from build123d import *

# Parameters (mm, degrees)
SKETCH1_W            = 133.35
SKETCH1_H            = 76.2
BOSS_EXTRUDE1_DEPTH  = 3
M2_CLEARANCE_HOLE1_D = 2.6
SKETCH7_R            = 3.75
SKETCH7_R_2          = 1.665
BOSS_EXTRUDE2_DEPTH  = 5.5
CUT_EXTRUDE1_DEPTH   = 77.989711163
FILLET1_R            = 5
SKETCH9_R            = 2.25
CUT_EXTRUDE2_DEPTH   = 1


with BuildPart() as part:
    # Sketch1 → Boss-Extrude1 (new body)
    with BuildSketch(Plane(origin=(0, 0, 0), x_dir=(0, 0, -1), z_dir=(1, 0, 0))):
        Rectangle(SKETCH1_W, SKETCH1_H)
    extrude(amount=BOSS_EXTRUDE1_DEPTH)

    # M2 Clearance Hole1 (through all)
    with Locations(Plane(origin=(3, 0, 0), x_dir=(0, 0, -1), z_dir=(1, 0, 0))):
        with Locations((-45, -30.1), (-45, 30.1), (42, 30.1), (42, -30.1)):
            Hole(M2_CLEARANCE_HOLE1_D / 2)

    # Sketch7 → Boss-Extrude2 (add)
    # profile 1 of 4: a face of its own
    with BuildSketch(Plane(origin=(3, 0, 0), x_dir=(0, 0, -1), z_dir=(1, 0, 0))):
        with Locations((-30.23150301, -26.854999996)):
            Circle(SKETCH7_R)
        with Locations((-30.23150301, -26.854999996)):
            Circle(SKETCH7_R_2, mode=Mode.SUBTRACT)
    # profile 2 of 4: a face of its own
    with BuildSketch(Plane(origin=(3, 0, 0), x_dir=(0, 0, -1), z_dir=(1, 0, 0))):
        with Locations((-30.23150301, 17.584000004)):
            Circle(SKETCH7_R)
        with Locations((-30.23150301, 17.584000004)):
            Circle(SKETCH7_R_2, mode=Mode.SUBTRACT)
    # profile 3 of 4: a face of its own
    with BuildSketch(Plane(origin=(3, 0, 0), x_dir=(0, 0, -1), z_dir=(1, 0, 0))):
        with Locations((52.82649699, 24.895000004)):
            Circle(SKETCH7_R)
        with Locations((52.82649699, 24.895000004)):
            Circle(SKETCH7_R_2, mode=Mode.SUBTRACT)
    # profile 4 of 4: a face of its own
    with BuildSketch(Plane(origin=(3, 0, 0), x_dir=(0, 0, -1), z_dir=(1, 0, 0))):
        with Locations((52.82649699, -34.162999996)):
            Circle(SKETCH7_R)
        with Locations((52.82649699, -34.162999996)):
            Circle(SKETCH7_R_2, mode=Mode.SUBTRACT)
    extrude(amount=BOSS_EXTRUDE2_DEPTH)

    # Sketch8 → Cut-Extrude1 (cut, through all)
    with BuildSketch(Plane(origin=(3, 0, 0), x_dir=(0, 0, -1), z_dir=(1, 0, 0))):
        Polygon((-51.675, -329.618471863), (-51.675, -38.1), (-51.675, 38.1), (-51.675, 329.618471863), (-634.711943726, 329.618471863), (-634.711943726, -329.618471863), align=None)
    extrude(amount=-CUT_EXTRUDE1_DEPTH, mode=Mode.SUBTRACT)

    # Fillet1
    fillet1_edges = [part.edges().sort_by_distance(p)[0] for p in [
        (1.5, -38.1, 51.675),
        (1.5, 38.1, 51.675),
        (1.5, -38.1, -66.675),
        (1.5, 38.1, -66.675),
    ]]
    fillet(fillet1_edges, radius=FILLET1_R)

    # Sketch9 → Cut-Extrude2 (cut)
    with BuildSketch(Plane(origin=(3, 0, 0), x_dir=(0, 0, -1), z_dir=(1, 0, 0))):
        with Locations((-45, -30.1)):
            Circle(SKETCH9_R)
        with Locations((-45, 30.1)):
            Circle(SKETCH9_R)
        with Locations((42, 30.1)):
            Circle(SKETCH9_R)
        with Locations((42, -30.1)):
            Circle(SKETCH9_R)
    extrude(amount=-CUT_EXTRUDE2_DEPTH, mode=Mode.SUBTRACT)


solid = part.part
Can you work these out from the model? Positions are in its coordinate system, mm. A direction names the side the tool comes from. Give positions to 0.01 mm unless a question says otherwise; leave off trailing zeros. Loops run counter-clockwise (first coordinate to the right, second up) from the corner with the lowest first, then second, coordinate; pieces in that order, holes last. Notation, with made-up numbers: (14.5, -24.75) -> (32.5, -24.75) arc R28 cw to (32.5, 5.25) -> close; hole circle Ø5 at (15.5, 77.25). An arc over 180 degrees is marked (long way). Write item = value, one per line.
1) Suppose I cut it at A-A on y = 30.1. Write out the boundary of the cut face in (x, z) (3 decimals).
Check result:
outline = (0, -66.675) -> (3, -66.675) -> (3, -44.25) -> (2, -44.25) -> (2, -43.3) -> (0, -43.3) -> close; (0, -40.7) -> (2, -40.7) -> (2, -39.75) -> (3, -39.75) -> (3, 42.75) -> (2, 42.75) -> (2, 43.7) -> (0, 43.7) -> close; (0, 46.3) -> (2, 46.3) -> (2, 47.25) -> (3, 47.25) -> (3, 51.675) -> (0, 51.675) -> close
2) Suppose I cut it at B-B on z = 45. Write out the boundary of the cut face in (x, y).
Check result:
outline = (0, -38.1) -> (3, -38.1) -> (3, -32.35) -> (2, -32.35) -> (2, -31.4) -> (0, -31.4) -> close; (0, -28.8) -> (2, -28.8) -> (2, -27.85) -> (3, -27.85) -> (3, 27.85) -> (2, 27.85) -> (2, 28.8) -> (0, 28.8) -> close; (0, 31.4) -> (2, 31.4) -> (2, 32.35) -> (3, 32.35) -> (3, 38.1) -> (0, 38.1) -> close
3) Suppose I cut it at C-C on x = 5.5. Give the number of separate pieces and of enclosed holes in the cut face, then the cut area to 3 significant figures.
Check result:
separate_pieces = 4
enclosed_holes = 4
area = 142 mm2
4) Suppose I cut it at D-D on z = 30.5. Write out the boundary of the cut face in (x, y).
Check result:
outline = (0, -38.1) -> (3, -38.1) -> (3, -30.6) -> (8.5, -30.6) -> (8.5, -28.5) -> (3, -28.5) -> (3, -25.21) -> (8.5, -25.21) -> (8.5, -23.11) -> (3, -23.11) -> (3, 13.84) -> (8.5, 13.84) -> (8.5, 15.94) -> (3, 15.94) -> (3, 19.23) -> (8.5, 19.23) -> (8.5, 21.32) -> (3, 21.32) -> (3, 38.1) -> (0, 38.1) -> close
5) I need wall thicknesses on L1, parallel to Y at x = 1.6, z = -42; L2, parallel to Y at x = 2.8, z = -42; L3, parallel to X at y = 11.5, z = -19. Which ranges of each line are inside material? Lowest first, please. Write a range as from..to.
Check result:
L1 = -38.1..-31.4, -28.8..28.8, 31.4..38.1
L2 = -38.1..-32.35, -27.85..27.85, 32.35..38.1
L3 = 0..3
6) Will these pins go through, and if not, where does the flat tip stop? pin 1 (3 mm diameter, centred on y = 17.58, z = 30.23, fed in from -X); pin 2 (1.7 mm diameter, centred on y = -27, z = 31, fed in from +X); pin 3 (2 mm diameter, centred on y = -30, z = -41, fed in from +X).
Check result:
pin_1 = 0
pin_2 = 3
pin_3 = 2
7) Thinking about a two-plate mould opening in Z: for faces 3 (the flat face through (1, 38.1, -7)), 4 (the cylindrical face through (0.99, 29.31, 43.97)), 5 (the cylindrical face through (1.479, -36.674, 50.171)), which applies, released by +Z, released by -Z, zero draft, split by the parting line, or undercut?
Check result:
face_3 = zero draft
face_4 = undercut
face_5 = released by +Z
8) For faces 1 (the cylindrical face through (5.712, -25.729, 26.655)), 2 (the cylindrical face through (1.521, -36.674, -65.171)), which set-ups out of +Z, -Z, +X, -X, +Y, -Y let a thin tool reach every point of the face, with its end or its side?
Check result:
face_1 = +X
face_2 = -Z, +X, -X, -Y
